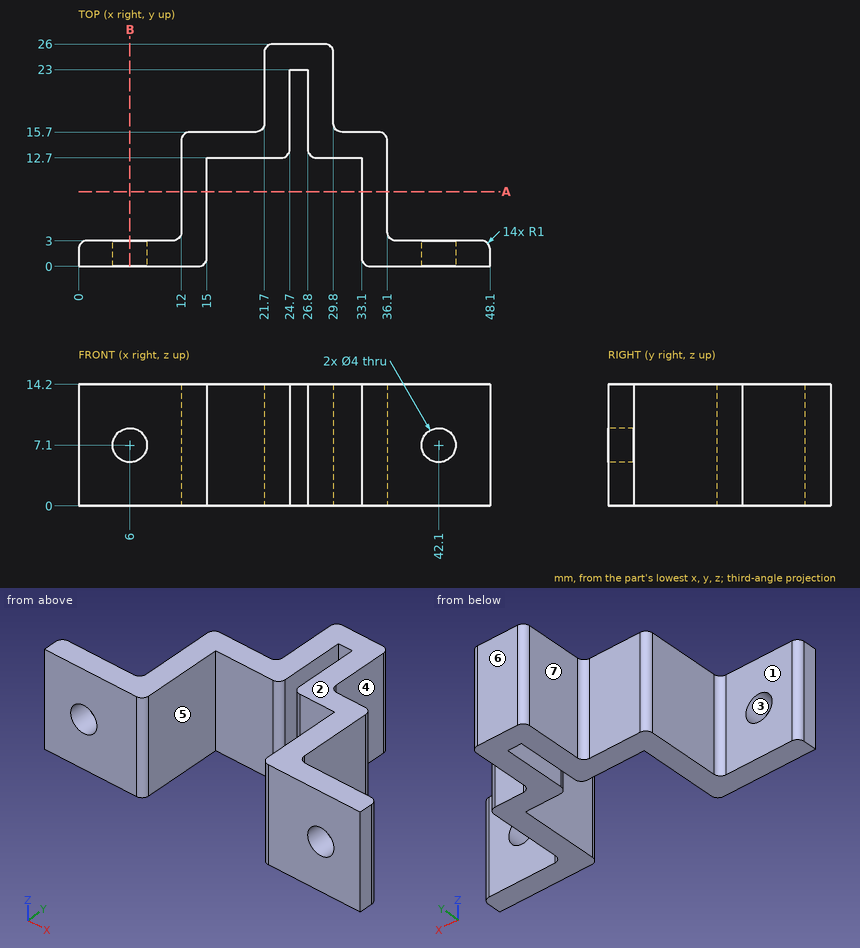
Check sheet for the drawn part. Datum: minimum x, y, z corner. Units: mm. A direction names the side the tool comes from. Give positions to 0.01 mm unless a question says otherwise; leave off trailing zeros. Order: outer loops, then holes, each group sorted by start corner. A loop starts at its lowest first (then second) coordinate and runs counter-clockwise, first axis right, second up.
1. Depth check by flat-ended pin: pin 1 (3.5 mm diameter, centred on x = 42.1, z = 7.1, fed in from -Y); pin 2 (10 mm diameter, centred on x = 18, y = 21, fed in from +Z); pin 3 (2.5 mm diameter, centred on y = 20.5, z = 7.5, fed in from -X); pin 4 (0.6 mm diameter, centred on x = 25.5, z = 6, fed in from -Y). Enter the tip coordinate at first touch or a pass-through.
Completed:
pin 1: passes through
pin 2: stops at z = 14.2
pin 3: stops at x = 21.7
pin 4: stops at y = 23
2. Draft check along Z on the marked faces 1, 2 and 3. Enter one of: pulls with the +Z half, pulls with the -Z half, needs draft (parallel to the pull), parting line crosses it, or undercut.
Completed:
face 1: needs draft
face 2: pulls with the +Z half
face 3: undercut
3. Scan lines: line 1 (Z direction, x = 6, y = 1.45); line 2 (X direction, y = 17.75, z = 11); line 3 (X direction, y = 14.25, z = 11.5). Record each from-to range of solid material in increasing order.
Completed:
line 1: z = 0 to 5.1, 9.1 to 14.2
line 2: x = 21.7 to 24.7, 26.8 to 29.8
line 3: x = 12 to 24.7, 26.8 to 36.1
4. Sectioned sample at B-B (x = 6). Record the boundary of the cut face in (y, z), then the cut area to 3 significant figures.
Completed:
outline: (0, 0) - (3, 0) - (3, 5.1) - (0, 5.1) - close; (0, 9.1) - (3, 9.1) - (3, 14.2) - (0, 14.2) - close
area: 30.6 mm2
5. Sectioned sample at A-A (y = 8.75). Record the boundary of the cut face in (x, z).
Completed:
outline: (12, 0) - (15, 0) - (15, 14.2) - (12, 14.2) - close; (33.1, 0) - (36.1, 0) - (36.1, 14.2) - (33.1, 14.2) - close
6. Access from +Z, -Z, +X, -X, +Y, -Y to the whole of each face (thin tool, end or side, straight path). Record for the marked faces 4, 5, 6 and 7.
Completed:
face 4: +Z, -Z, +X, +Y
face 5: +Z, -Z, -Y
face 6: +Z, -Z, +X, -X, +Y
face 7: +Z, -Z, -X, +Y
